```python
from build123d import *

# Parameters (mm, degrees)
F0_W     = 25.4
F0_H     = 31.75
F1_DEPTH = 38.1
F3_DEPTH = 25.908


with BuildPart() as f1:
    # F0 (on Right) → F1 (new body)
    with BuildSketch(Plane.YZ):
        with Locations((12.7, 15.875)):
            Rectangle(F0_W, F0_H)
    extrude(amount=F1_DEPTH)

    # F2 (on face) → F3 (join)
    with BuildSketch(Plane.YZ.offset(38.1)):
        Polygon((25.4, 31.75), (19.762445, 31.75), (0, 5.154566), (0, 0), (25.4, 0), align=None)
    extrude(amount=F3_DEPTH)


solid = f1.part
```
Here's how the part is built. I have some questions about the finished solid (model axes, mm). A direction names the side the tool comes from. Give positions to 0.01 mm unless a question says otherwise; leave off trailing zeros. Order: outer loops, then holes, each group sorted by start corner. A loop starts at its lowest first (then second) coordinate and runs counter-clockwise, first axis right, second up. Notation, with made-up numbers: (57.25, 75) - (62.25, 75) arc R17 ccw to (62.25, 95) - close; hole circle Ø4 at (37.5, -5.75). An arc over 180 degrees is marked (long way). Answer as a JSON object with one key per item and string values. Group by question number.
Item 1: Which directions (+Z, -Z, +X, -X, +Y, -Y) give clear straight access to the entire face, cutting with the end or side of a thin tool? Please do faces 1 (the flat face through (0, 13, 16)), 2 (the flat face through (38.1, 8, 22)).
Item 2: For P1, Ø6, axis at x = 54.5, z = 20.5, coming from the -Y side, with a flat end and sliding along its axis, tell me the tip position at first contact or that it passes through.
Item 3: If we section it at A-A on x = 60.5: Please give me the cut outline in (y, z), and give its area (3 significant figures).
Item 4: Please list where these lines run through material, in increasing order: probe 1 along X at (y, z) = (17.25, 30); probe 2 along Z at (x, y) = (46, 7.5); probe 3 along Y at (x, z) = (45, 18).
Item 5: If we section it at B-B on y = 2: Please give me the cut outline in (x, z), and give its area (3 significant figures).
Item 6: If we section it at C-C on z = 15: Please give me the cut outline in (x, y).
Result set:
{
 "1": {"face 1": "+Z, -Z, -X, +Y, -Y", "face 2": "+Z, +X, -Y"},
 "2": {"P1": "y = 9.17"},
 "3": {"outline": "(0, 0) - (25.4, 0) - (25.4, 31.75) - (19.76, 31.75) - (0, 5.15) - close", "area": "544 mm²"},
 "4": {"probe 1": "0 to 38.1", "probe 2": "0 to 15.25", "probe 3": "9.55 to 25.4"},
 "5": {"outline": "(0, 0) - (64.01, 0) - (64.01, 7.85) - (38.1, 7.85) - (38.1, 31.75) - (0, 31.75) - close", "area": "1,410 mm²"},
 "6": {"outline": "(0, 0) - (38.1, 0) - (38.1, 7.32) - (64.01, 7.32) - (64.01, 25.4) - (0, 25.4) - close"}
}
